Source: CAD feature listing. Evaluate the final solid. Frame: model axes, mm. Face numbers are marked on the shaded views. A direction names the side the tool comes from. Give positions to 0.01 mm unless a question says otherwise; leave off trailing zeros. Loops run counter-clockwise (first coordinate to the right, second up) from the corner with the lowest first, then second, coordinate; pieces in that order, holes last. Notation, with made-up numbers: (16, -38.5) -> (39, -38.5) arc R14 cw to (39, -30.5) -> close; hole circle Ø2 at (-27, 7). An arc over 180 degrees is marked (long way). Answer as a JSON object with one key per item and string values. Group by question number.
from build123d import *

# Parameters (mm, degrees)
F0_W      = 50
F0_H      = 40
F1_DEPTH  = 20
F2_W      = 48
F2_H      = 38
F3_DEPTH  = 19
F4_W      = 5
F4_H      = 5
F5_DEPTH  = 19
F6_R      = 1.5
F7_DEPTH  = 10
F8_R      = 2.5
F8_R_2    = 1.5
F9_DEPTH  = 5
F10_DEPTH = 2
F11_R     = 5
F11_R_2   = 2.5
F12_DEPTH = 2
F13_R     = 1.5
F14_DEPTH = 2


with BuildPart() as f1:
    # F0 (on Top) → F1 (new body)
    with BuildSketch(Plane.XY):
        with Locations((-30.7756610087, 24.588953238)):
            Rectangle(F0_W, F0_H)
    extrude(amount=F1_DEPTH)

    # F2 (on face) → F3 (cut)
    with BuildSketch(Plane.XY.offset(20)):
        with Locations((-30.7756610087, 24.588953238)):
            Rectangle(F2_W, F2_H)
    extrude(amount=-F3_DEPTH, mode=Mode.SUBTRACT)

    # F4 (on face) → F5 (join)
    with BuildSketch(Plane.XY.offset(1)):
        with Locations((-52.2756610087, 41.088953238)):
            Rectangle(F4_W, F4_H)
        with Locations((-9.2756610087, 41.088953238)):
            Rectangle(F4_W, F4_H)
        with Locations((-9.2756610087, 8.088953238)):
            Rectangle(F4_W, F4_H)
        with Locations((-52.2756610087, 8.088953238)):
            Rectangle(F4_W, F4_H)
    extrude(amount=F5_DEPTH)

    # F6 (on face) → F7 (cut)
    with BuildSketch(Plane.XY.offset(20)):
        with Locations((-52.2756610087, 8.088953238)):
            Circle(F6_R)
        with Locations((-52.2756610087, 41.088953238)):
            Circle(F6_R)
        with Locations((-9.2756610087, 41.088953238)):
            Circle(F6_R)
        with Locations((-9.2756610087, 8.088953238)):
            Circle(F6_R)
    extrude(amount=-F7_DEPTH, mode=Mode.SUBTRACT)

    # F8 (on face) → F9 (join)
    with BuildSketch(Plane.XY.offset(1)):
        with Locations((-33.7756610087, 20.588953238)):
            Circle(F8_R)
        with Locations((-33.7756610087, 20.588953238)):
            Circle(F8_R_2, mode=Mode.SUBTRACT)
        with Locations((-18.7756610087, 30.588953238)):
            Circle(F8_R)
        with Locations((-18.7756610087, 30.588953238)):
            Circle(F8_R_2, mode=Mode.SUBTRACT)
    extrude(amount=F9_DEPTH)

    # F10 (cut): faces of the model
    f10_faces = [f1.faces().sort_by_distance(p)[0] for p in [
        (-33.7756610087, 20.588953238, 1),
        (-18.7756610087, 30.588953238, 1),
    ]]
    extrude(f10_faces, amount=-F10_DEPTH, mode=Mode.SUBTRACT)

    # F11 (on face) → F12 (join)
    with BuildSketch(Plane.XY.offset(1)):
        with Locations((-18.7756610087, 30.588953238)):
            Circle(F11_R)
        with Locations((-18.7756610087, 30.588953238)):
            Circle(F11_R_2, mode=Mode.SUBTRACT)
        with Locations((-33.7756610087, 20.588953238)):
            Circle(F11_R)
        with Locations((-33.7756610087, 20.588953238)):
            Circle(F11_R_2, mode=Mode.SUBTRACT)
    extrude(amount=F12_DEPTH)

    # F13 (on face) → F14 (cut)
    with BuildSketch(Plane(origin=(0, 0, 0), x_dir=(1, 0, 0), z_dir=(0, 0, -1))):
        Polygon((-16.1775847973, -32.088953238), (-16.1775847973, -29.088953238), (-18.7756610087, -27.588953238), (-21.37373722, -29.088953238), (-21.37373722, -32.088953238), (-18.7756610087, -33.588953238), align=None)
        with Locations((-18.7756610087, -30.588953238)):
            Circle(F13_R, mode=Mode.SUBTRACT)
        Polygon((-31.2851968259, -22.0268234043), (-31.2851968259, -19.1510830716), (-33.7756610087, -17.7132129053), (-36.2661251915, -19.1510830716), (-36.2661251915, -22.0268234043), (-33.7756610087, -23.4646935706), align=None)
        with Locations((-33.7756610087, -20.588953238)):
            Circle(F13_R, mode=Mode.SUBTRACT)
    extrude(amount=-F14_DEPTH, mode=Mode.SUBTRACT)


solid = f1.part
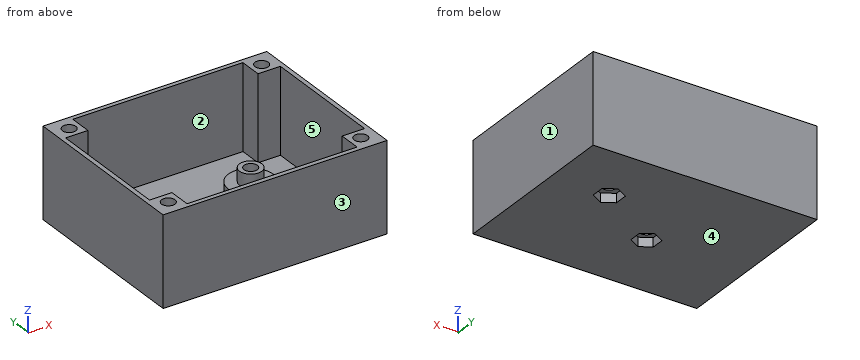
(1) Material intervals for line 1 (X direction, y = 28, z = 10.5); line 2 (Y direction, x = -19, z = 10); line 3 (Y direction, x = -18, z = 1.25), sorted ascending. Write a range as from..to.
(2) Mould query, pull axis Y, two halves, no side actions, for the marked faces 3, 4 and 5. Classes: pulls with the +Y half, pulls with the -Y half, needs draft (parallel to the pull), parting line crosses it, or undercut.
(3) Section query C-C on y = 36.5. Return the cut outline in (x, z), plus the area to 3 significant figures.
(4) Section query D-D on y = 25. Return the cut outline in (x, z), plus the area to 3 significant figures.
(5) Section query B-B on x = -43.5. Return the cut outline in (y, z).
(6) First-contact query: pin 1 (10 mm diameter, centred on x = -33.5, y = 29, fed in from +Z); pin 2 (11.5 mm diameter, centred on x = -29, y = 20.5, fed in from +Z); pin 3 (2.5 mm diameter, centred on x = -17.5, y = 30, fed in from -Z). Flat tips, straight axial feed; report the tip coordinate or a pass-through.
(7) Access query for the marked faces 1 and 2. Directions: +Z, -Z, +X, -X, +Y, -Y. A direction counts if a zero-diameter tool reaches every point of the face in a straight line with its end or side. Return the directions, or none.
(8) Section query A-A on z = 11. Return the cut outline in (x, y), plus the area to 3 significant figures.
Result:
{
 "1": {"line 1": "-55.78..-54.78, -6.78..-5.78", "line 2": "4.59..5.59, 43.59..44.59", "line 3": "4.59..5.59, 25.65..28.04, 33.14..35.53, 43.59..44.59"},
 "2": {"face 3": "pulls with the -Y half", "face 4": "needs draft", "face 5": "undercut"},
 "3": {"outline": "(-55.78, 0) -> (-5.78, 0) -> (-5.78, 20) -> (-6.78, 20) -> (-6.78, 1) -> (-54.78, 1) -> (-54.78, 20) -> (-55.78, 20) -> close", "area": "88.0 mm²"},
 "4": {"outline": "(-55.78, 0) -> (-5.78, 0) -> (-5.78, 20) -> (-6.78, 20) -> (-6.78, 1) -> (-31.42, 1) -> (-31.42, 3) -> (-36.13, 3) -> (-36.13, 1) -> (-54.78, 1) -> (-54.78, 20) -> (-55.78, 20) -> close", "area": "97.4 mm²"},
 "5": {"outline": "(4.59, 0) -> (44.59, 0) -> (44.59, 20) -> (43.59, 20) -> (43.59, 1) -> (5.59, 1) -> (5.59, 20) -> (4.59, 20) -> close"},
 "6": {"pin 1": "z = 3", "pin 2": "z = 6", "pin 3": "z = 2"},
 "7": {"face 1": "+Z, -Z, +X, +Y, -Y", "face 2": "+Z"},
 "8": {"outline": "(-55.78, 4.59) -> (-5.78, 4.59) -> (-5.78, 44.59) -> (-55.78, 44.59) -> close; hole (-54.78, 10.59) -> (-49.78, 10.59) -> (-49.78, 5.59) -> (-11.78, 5.59) -> (-11.78, 10.59) -> (-6.78, 10.59) -> (-6.78, 38.59) -> (-11.78, 38.59) -> (-11.78, 43.59) -> (-49.78, 43.59) -> (-49.78, 38.59) -> (-54.78, 38.59) -> close; hole circle Ø3 at (-52.28, 8.09); hole circle Ø3 at (-52.28, 41.09); hole circle Ø3 at (-9.28, 8.09); hole circle Ø3 at (-9.28, 41.09)", "area": "248 mm²"}
}
